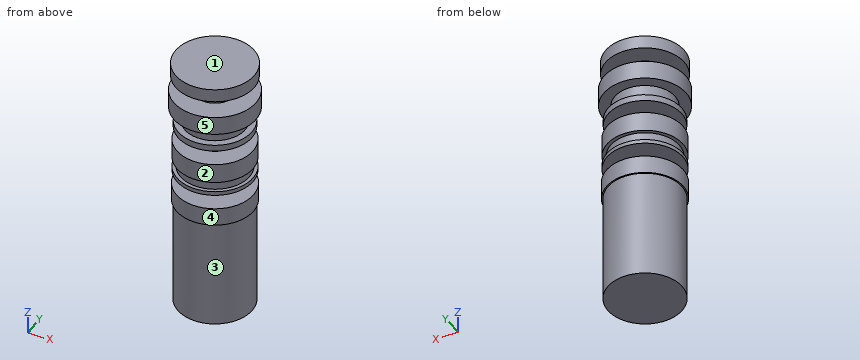
from build123d import *

# Parameters (mm, degrees)
F0_W   = 10.3888958693
F0_H   = 8.3731412888
F0_W_2 = 15.6360119581
F0_H_2 = 7.9048592597
F0_W_3 = 9.6391905099
F0_H_3 = 7.3461066931
F0_W_4 = 17.8349073976
F0_H_4 = 5.2964619827
F0_W_5 = 9.5420926809
F0_H_5 = 7.5158830732
F0_W_6 = 19.2370712757
F0_H_6 = 42.4508359283
F0_H_7 = 14.6481841803


with BuildPart() as f1:
    # F0 (on Front) → F1 (revolve)
    with BuildSketch(Plane.XZ):
        Polygon((0, 54.1152916849), (0, 60.9378516674), (-20.3126184642, 60.9378516674), (-20.3126184642, 54.1152916849), (-10.3888958693, 54.1152916849), align=None)
        with Locations((-5.1944479346, 49.9287210405)):
            Rectangle(F0_W, F0_H)
        Polygon((0, 36.1285470426), (0, 45.7421503961), (-10.3888958693, 45.7421503961), (-21.2429668754, 45.7421503961), (-21.2429668754, 36.1285470426), (-15.6360119581, 36.1285470426), align=None)
        with Locations((-7.8180059791, 32.1761174127)):
            Rectangle(F0_W_2, F0_H_2)
        Polygon((0, 24.9254349619), (0, 28.2236877829), (-15.6360119581, 28.2236877829), (-19.0841853619, 28.2236877829), (-19.0841853619, 24.9254349619), (-9.6391905099, 24.9254349619), align=None)
        with Locations((-4.819595255, 21.2523816153)):
            Rectangle(F0_W_3, F0_H_3)
        Polygon((0, 7.384730503), (0, 17.5793282688), (-9.6391905099, 17.5793282688), (-19.6838658303, 17.5793282688), (-19.6838658303, 7.384730503), (-17.8349073976, 7.384730503), align=None)
        with Locations((-8.9174536988, 4.7364995116)):
            Rectangle(F0_W_4, F0_H_4)
        Polygon((1.2327310396, 2.0882685203), (0, 2.0882685203), (-17.8349073976, 2.0882685203), (-19.6838658303, 2.0882685203), (-19.6838658303, 0), (-9.5420926809, 0), (0, 0), (1.2327310396, 0), align=None)
        with Locations((-4.7710463405, -3.7579415366)):
            Rectangle(F0_W_5, F0_H_5)
        Polygon((0, -16.8938729912), (0, -7.5158830732), (-9.5420926809, -7.5158830732), (-19.9061166495, -7.5158830732), (-19.9061166495, -16.8938729912), (-19.2370712757, -16.8938729912), align=None)
        with Locations((-9.6185356379, -38.1192909554)):
            Rectangle(F0_W_6, F0_H_6)
        with Locations((-9.6185356379, -66.6688010097)):
            Rectangle(F0_W_6, F0_H_7)
    revolve(axis=Axis((0, 0, -38.1192909554), (0, 0, -1)))


solid = f1.part
CAD build for the part. Positions are in the model's coordinates, mm. Face numbers are marked on the shaded views. A direction names the side the tool comes from. Coordinates: 2 decimals unless noted, no trailing zeros. Order: outer loops, then holes, each group sorted by start corner. A loop starts at its lowest first (then second) coordinate and runs counter-clockwise, first axis right, second up. Notation, with made-up numbers: (-29, 76.5) -> (-9, 76.5) arc R24 cw to (-9, 103.5) -> close; hole circle Ø10 at (-39, -5.75). An arc over 180 degrees is marked (long way). Answer in a Markdown table with one row per item.
1) Band-saw the part on A-A (z = -18.5). List the corners of the cut face in (x, y).
Check values:
| item | result |
|---|---|
| outline | circle Ø38.47 at (0, 0) |
2) Flat gauge pins, fed straight in: P1, Ø4, axis at x = 3, z = -8, coming from the -Y side; P2, Ø1, axis at x = 2, z = 24.5, coming from the +Y side; P3, Ø10, axis at y = 6.5, z = -32.5, coming from the -X side. Where does each tip first touch, or does it go through?
Check values:
| item | result |
|---|---|
| P1 | y = -19.88 |
| P2 | y = 19 |
| P3 | x = -19.18 |
3) Drill centre lines: line 1 (Z direction, x = -9, y = -4); line 2 (Z direction, x = -12, y = 14); line 3 (Z direction, x = -10.5, y = -6). Where is each one in solid material? Low to high.
Check values:
| item | result |
|---|---|
| line 1 | -73.99 to -7.52, 0 to 17.58, 24.93 to 60.94 |
| line 2 | -73.99 to -7.52, 0 to 2.09, 7.38 to 17.58, 24.93 to 28.22, 36.13 to 45.74, 54.12 to 60.94 |
| line 3 | -73.99 to -7.52, 0 to 17.58, 24.93 to 45.74, 54.12 to 60.94 |
4) Band-saw the part on B-B (x = -13). Give the number of separate pieces and of enclosed holes in the cut face, and give its area (3 significant figures).
Check values:
| item | result |
|---|---|
| separate pieces | 4 |
| enclosed holes | 0 |
| area | 3,160 mm2 |
5) Mould opens along Z. For the marked faces 1, 2 and 3 say: pulls with the +Z half, pulls with the -Z half, needs draft (parallel to the pull), parting line crosses it, or undercut.
Check values:
| item | result |
|---|---|
| face 1 | pulls with the +Z half |
| face 2 | undercut |
| face 3 | needs draft |
6) Which spindle directions (+Z, -Z, +X, -X, +Y, -Y) get a long thin tool onto all of the face, cutting with end or side? Do the marked faces 4 and 5. Say none if no direction does.
Check values:
| item | result |
|---|---|
| face 4 | -Z |
| face 5 | +Z, -Z |
